For this review, take the finished solid that the model builds, in its own axes (mm). A direction names the side the tool comes from. Give positions to 0.01 mm unless a question says otherwise; leave off trailing zeros. Order: outer loops, then holes, each group sorted by start corner. A loop starts at its lowest first (then second) coordinate and runs counter-clockwise, first axis right, second up.
Item 1: Consider section A-A (x = 66.5). Give the boundary of the cut face in (y, z), plus the area to 4 significant figures.
Item 2: Consider section C-C (y = 3.95). Give the number of separate pieces and of enclosed holes in the cut face, plus the area to 3 significant figures.
Item 3: For probe 1 along X at (y, z) = (2.9, -39) (3 decimals); probe 2 along Z at (x, y) = (66.5, 1.35); probe 3 along X at (y, z) = (2.15, -35.5), list the stretches that pass through material, from the lowest coordinate up.
Item 4: For P1, Ø1, axis at x = 101.5, y = 4, coming from the +Z side; P2, Ø3, axis at y = 2, z = 1, coming from the -X side; P3, Ø5, axis at x = 6, z = -44.5, coming from the -Y side, all flat-tipped, find the tip position at first contact; note any pin that passes through.
Item 5: Machinability: for faces 1 (the flat face through (125, 2, -7)), 2 (the cylindrical face through (16.97, 2.46, -39.92)), 3 (the flat face through (125, 2, -43)), which of the approach directions +Z, -Z, +X, -X, +Y, -Y give a long, thin tool a straight path to every point of the face, cutting with its end or side? Answer none if there is none.
Item 6: Consider section D-D (x = 110). Give the boundary of the cut face in (y, z), plus the area to 4 significant figures.
Item 7: The part is to be moulded in two halves that separate along Z. For faces 4 (the flat face through (26, 3, 2.5)), 5 (the cylindrical face through (124.74, 2.46, -35.66)), 6 (the cylindrical face through (123.5, 2.54, -49.07)), say which applies: released by +Z, released by -Z, zero draft, split by the parting line, or undercut.
Item 8: Consider section B-B (z = -15). Give the boundary of the cut face in (x, y), plus the area to 4 significant figures.
```python
from build123d import *

# Parameters (mm, degrees)
SKETCH1_W           = 125
SKETCH1_H           = 50.5
SKETCH1_R           = 1.25
SKETCH1_R_2         = 2
BOSS_EXTRUDE1_DEPTH = 5
FILLET1_R           = 5
CHAMFER1_SIZE       = 1.5
SKETCH3_W           = 3
SKETCH3_H           = 32.5
SKETCH3_W_2         = 26
SKETCH3_H_2         = 3
BOSS_EXTRUDE2_DEPTH = 5
SKETCH5_W           = 26
SKETCH5_H           = 5
CUT_EXTRUDE1_DEPTH  = 0.5
SKETCH6_W           = 32.5
SKETCH6_H           = 5
BOSS_EXTRUDE4_DEPTH = 0.5


with BuildPart() as part:
    # Sketch1 → Boss-Extrude1 (new body)
    with BuildSketch(Plane(origin=(0, 0, 0), x_dir=(1, 0, 0), z_dir=(0, 1, 0))):
        with Locations((62.5, 25.25)):
            Rectangle(SKETCH1_W, SKETCH1_H)
        with Locations(Location((16.5, 1.5, 0), (0, 0, 270))):
            Circle(SKETCH1_R, mode=Mode.SUBTRACT)
        with Locations(Location((6, 6, 0), (0, 0, 270))):
            Circle(SKETCH1_R_2, mode=Mode.SUBTRACT)
        with Locations(Location((36.5, 1.5, 0), (0, 0, 270))):
            Circle(SKETCH1_R, mode=Mode.SUBTRACT)
        with Locations(Location((119, 6, 0), (0, 0, 270))):
            Circle(SKETCH1_R_2, mode=Mode.SUBTRACT)
        with Locations(Location((16.125, 39, 0), (0, 0, 270))):
            Circle(SKETCH1_R, mode=Mode.SUBTRACT)
        with Locations(Location((6, 44.5, 0), (0, 0, 270))):
            Circle(SKETCH1_R_2, mode=Mode.SUBTRACT)
        with Locations(Location((36.875, 39, 0), (0, 0, 270))):
            Circle(SKETCH1_R, mode=Mode.SUBTRACT)
        with Locations(Location((66.5, 35.5, 0), (0, 0, 270))):
            Circle(SKETCH1_R, mode=Mode.SUBTRACT)
        with Locations(Location((123.5, 35.5, 0), (0, 0, 270))):
            Circle(SKETCH1_R, mode=Mode.SUBTRACT)
        with Locations(Location((66.5, 15, 0), (0, 0, 270))):
            Circle(SKETCH1_R, mode=Mode.SUBTRACT)
        with Locations(Location((123.5, 15, 0), (0, 0, 270))):
            Circle(SKETCH1_R, mode=Mode.SUBTRACT)
        with Locations(Location((119, 44.5, 0), (0, 0, 270))):
            Circle(SKETCH1_R_2, mode=Mode.SUBTRACT)
    extrude(amount=BOSS_EXTRUDE1_DEPTH)

    # Fillet1
    fillet1_edges = [part.edges().sort_by_distance(p)[0] for p in [
        (125, 2.5, 0),
        (0, 2.5, 0),
        (0, 2.5, -50.5),
        (125, 2.5, -50.5),
    ]]
    fillet(fillet1_edges, radius=FILLET1_R)

    # Chamfer1
    chamfer1_edges = [part.edges().sort_by_distance(p)[0] for p in [
        (119, 0, -8),
        (6, 0, -8),
        (6, 0, -46.5),
        (119, 0, -46.5),
    ]]
    chamfer(chamfer1_edges, length=CHAMFER1_SIZE)

    # Sketch3 → Boss-Extrude2 (add)
    with BuildSketch(Plane(origin=(0, 5, 0), x_dir=(1, 0, 0), z_dir=(0, 1, 0))):
        with Locations((126.5, 25.25)):
            Rectangle(SKETCH3_W, SKETCH3_H)
        with Locations((26.5, -1.5)):
            Rectangle(SKETCH3_W_2, SKETCH3_H_2)
    extrude(amount=-BOSS_EXTRUDE2_DEPTH)

    # Sketch5 → Cut-Extrude1 (cut)
    with BuildSketch(Plane.XY.offset(3)):
        with Locations((26.5, 2.5)):
            Rectangle(SKETCH5_W, SKETCH5_H)
    extrude(amount=-CUT_EXTRUDE1_DEPTH, mode=Mode.SUBTRACT)

    # Sketch6 → Boss-Extrude4 (add)
    with BuildSketch(Plane(origin=(128, 0, 0), x_dir=(0, 0, -1), z_dir=(1, 0, 0))):
        with Locations((25.25, 2.5)):
            Rectangle(SKETCH6_W, SKETCH6_H)
    extrude(amount=BOSS_EXTRUDE4_DEPTH)


solid = part.part
```
Resolved:
1. outline: (0, -50.5) - (5, -50.5) - (5, -36.75) - (0, -36.75) - close; (0, -34.25) - (5, -34.25) - (5, -16.25) - (0, -16.25) - close; (0, -13.75) - (5, -13.75) - (5, 0) - (0, 0) - close
1. area: 227.5 mm2
2. separate pieces: 1
2. enclosed holes: 12
2. area: 6,380 mm2
3. probe 1: x = 0 to 14.875, 17.375 to 35.625, 38.125 to 128.5
3. probe 2: z = -50.5 to -36.75, -34.25 to -16.25, -13.75 to 0
3. probe 3: x = 0 to 65.25, 67.75 to 122.25, 124.75 to 128.5
4. P1: stops at z = 0
4. P2: stops at x = 2.82
4. P3: stops at y = 1
5. face 1: +Z, +X, +Y, -Y
5. face 2: +Y, -Y
5. face 3: -Z, +X, +Y, -Y
6. outline: (0, -50.5) - (5, -50.5) - (5, 0) - (0, 0) - close
6. area: 252.5 mm2
7. face 4: released by +Z
7. face 5: undercut
7. face 6: released by -Z
8. outline: (0, 0) - (65.25, 0) - (65.25, 5) - (0, 5) - close; (67.75, 0) - (122.25, 0) - (122.25, 5) - (67.75, 5) - close; (124.75, 0) - (128.5, 0) - (128.5, 5) - (124.75, 5) - close
8. area: 617.5 mm2
